The drawing under review shows one solid part. Ordinate dimensions are in mm from its lowest x, y, z. A direction names the side the tool comes from. Coordinates: 2 decimals unless noted, no trailing zeros. Order: outer loops, then holes, each group sorted by start corner. A loop starts at its lowest first (then second) coordinate and runs counter-clockwise, first axis right, second up.
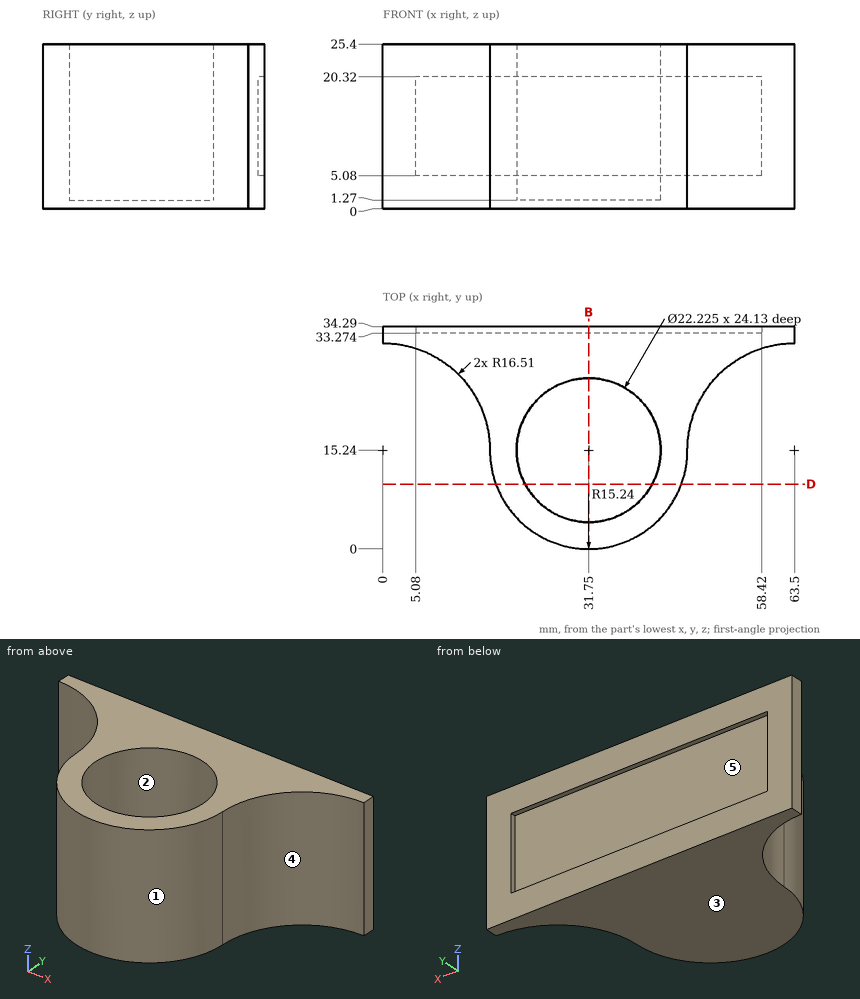
(1) Draft analysis for pull direction Z (two halves, no side actions). For the marked faces 3, 4 and 5, state which applies: released by +Z, released by -Z, zero draft, split by the parting line, or undercut.
A:
face 3: released by -Z
face 4: zero draft
face 5: undercut
(2) We need section D-D, the plane y = 10. Write out the cut boundary in (x, z).
A:
outline: (17.44, 0) - (46.06, 0) - (46.06, 25.4) - (41.55, 25.4) - (41.55, 1.27) - (21.95, 1.27) - (21.95, 25.4) - (17.44, 25.4) - close
(3) Machinability: for the marked faces 1 and 2, which of the approach directions +Z, -Z, +X, -X, +Y, -Y give a long, thin tool a straight path to every point of the face, cutting with its end or side? Answer none if there is none.
A:
face 1: +Z, -Z, -Y
face 2: +Z
(4) Wall thickness on probe 1 along Y at (x, z) = (31.75, 16.5); probe 2 along X at (y, z) = (15.5, 18.5); probe 3 along Y at (x, z) = (25.5, 3.5): over which ranges is each line inside the solid? List them lowest first.
A:
probe 1: y = 0 to 4.13, 26.35 to 33.27
probe 2: x = 16.51 to 20.64, 42.86 to 46.99
probe 3: y = 1.34 to 6.05, 24.43 to 34.29
(5) For pin 1 Ø1 at (x, y) = (44.5, 11.5) entering from -Z; pin 2 Ø8 at (x, z) = (55, 17.5) entering from -Y; pin 3 Ø4 at (x, z) = (53, 15.5) entering from +Y; pin 4 Ø4 at (y, z) = (7.5, 3.5) entering from -X, all flat-tipped, find the tip position at first contact; note any pin that passes through.
A:
pin 1: stops at z = 0
pin 2: stops at y = 26.03
pin 3: stops at y = 33.27
pin 4: stops at x = 17.63
(6) We need section B-B, the plane x = 31.75. Write out the cut boundary in (y, z).
A:
outline: (0, 0) - (34.29, 0) - (34.29, 5.08) - (33.27, 5.08) - (33.27, 20.32) - (34.29, 20.32) - (34.29, 25.4) - (26.35, 25.4) - (26.35, 1.27) - (4.13, 1.27) - (4.13, 25.4) - (0, 25.4) - close
